Verification items for the finished model (mm, model axes). Face numbers are marked on the shaded views. A direction names the side the tool comes from. Round coordinates to 2 decimals unless told otherwise and drop trailing zeros. Write each loop counter-clockwise with the first axis right and the second up, starting at its lowest first coordinate (ties: lowest second). Pieces come first, ordered by that corner, then holes. Notation, with made-up numbers: M 22,26.25 L 76,26.25 A21 ccw 76,34.25 Z; hole C 12.25,-3 d9. An arc over 180 degrees is marked long. One line per question, with ' | ' between items.
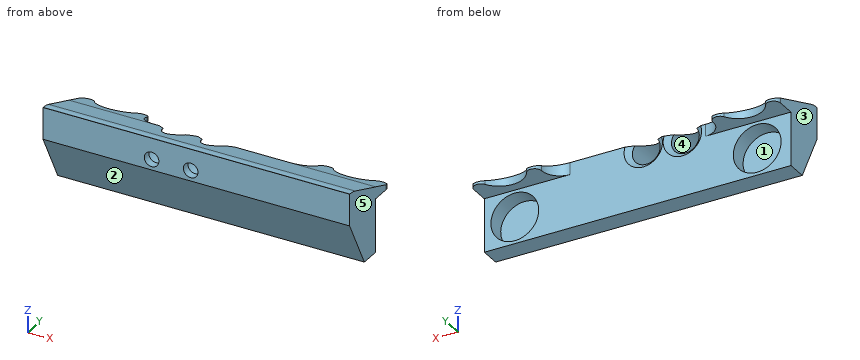
from build123d import *

# Parameters (mm, degrees)
SKETCH1_W               = 115.75
SKETCH1_H               = 30.5
SKETCH1_R               = 2.75
SKETCH1_R_2             = 9.025
BOSS_EXTRUDE1_DEPTH     = 17.25
SKETCH3_R               = 9.025
BOSS_EXTRUDE2_DEPTH     = 10.75
SKETCH4_R               = 5.25
CUT_EXTRUDE1_DEPTH      = 14.25
CUT_EXTRUDE2_DEPTH      = 120.171619944
CUT_EXTRUDE2_DEPTH_BACK = 120.171619944
BOSS_EXTRUDE4_REACH     = 67.617
CHAMFER1_SIZE           = 2


with BuildPart() as part:
    # Sketch1 → Boss-Extrude1 (new body)
    with BuildSketch(Plane(origin=(0, 0, 0), x_dir=(1, 0, 0), z_dir=(0, 1, 0))):
        with Locations((2.125, 7.25)):
            Rectangle(SKETCH1_W, SKETCH1_H)
        with Locations(Location((0, 0, 0), (0, 0, 270))):
            Circle(SKETCH1_R, mode=Mode.SUBTRACT)
        with Locations(Location((-14.75, 0, 0), (0, 0, 270))):
            Circle(SKETCH1_R, mode=Mode.SUBTRACT)
        with Locations(Location((48.5, 12.4, 0), (0, 0, 270))):
            Circle(SKETCH1_R_2, mode=Mode.SUBTRACT)
        with Locations(Location((-43, 12.4, 0), (0, 0, 270))):
            Circle(SKETCH1_R_2, mode=Mode.SUBTRACT)
    extrude(amount=BOSS_EXTRUDE1_DEPTH)

    # Sketch3 → Boss-Extrude2 (add)
    with BuildSketch(Plane.XZ):
        with Locations(Location((48.5, -12.4, 0), (0, 0, 270))):
            Circle(SKETCH3_R)
        with Locations(Location((-43, -12.4, 0), (0, 0, 270))):
            Circle(SKETCH3_R)
    extrude(amount=-BOSS_EXTRUDE2_DEPTH)

    # Sketch4 → Cut-Extrude1 (cut)
    with BuildSketch(Plane(origin=(0, 17.25, 0), x_dir=(1, 0, 0), z_dir=(0, 1, 0))):
        with Locations(Location((-14.75, 0, 0), (0, 0, 270))):
            Circle(SKETCH4_R)
        with Locations(Location((0, 0, 0), (0, 0, 270))):
            Circle(SKETCH4_R)
    extrude(amount=-CUT_EXTRUDE1_DEPTH, mode=Mode.SUBTRACT)

    # Sketch8 → Cut-Extrude2 (cut, two sides: drawn at the far end of the back side and taken through both)
    with BuildSketch(Plane(origin=(60, 0, 0), x_dir=(0, 0, -1), z_dir=(1, 0, 0)).offset(-CUT_EXTRUDE2_DEPTH_BACK)):
        with BuildLine():
            Line((-2.2, 17.25), (-7.34681784, 3.717418611))
            ThreePointArc((-7.34681784, 3.717418611), (-7.835348962, 1.969746414), (-8, 0.162563302))
            Line((-8, 0.162563302), (-8, 17.25))
            Line((-8, 17.25), (-2.2, 17.25))
        make_face()
        Polygon((22.5, 9.75), (4, 0), (22.5, 0), align=None)
    extrude(amount=CUT_EXTRUDE2_DEPTH + CUT_EXTRUDE2_DEPTH_BACK, mode=Mode.SUBTRACT)

    # Boss-Extrude4: up to this plane
    boss_extrude4_end = Plane(origin=(-55.75, 17.25, 2.2), z_dir=(0, -0.35548553095217983, -0.9346817839690934))
    # Sketch7 → Boss-Extrude4 (add, up to the surface)
    with BuildSketch(Plane.XY.offset(-2.3), mode=Mode.PRIVATE) as boss_extrude4_sk1:
        with BuildLine():
            ThreePointArc((39.434120731, 25.3875), (36.45982129, 26.619495167), (34.5, 24.065406335))
            ThreePointArc((34.5, 24.065406335), (32.503813701, 19.246186299), (27.684593665, 17.25))
            Line((27.684593665, 17.25), (60, 17.25))
            Line((60, 17.25), (60, 24.065406335))
            ThreePointArc((60, 24.065406335), (58.04017871, 26.619495167), (55.065879269, 25.3875))
            ThreePointArc((55.065879269, 25.3875), (47.25, 20.875), (39.434120731, 25.3875))
        make_face()
    boss_extrude4_tool1 = split(extrude(boss_extrude4_sk1.sketch, amount=BOSS_EXTRUDE4_REACH, mode=Mode.PRIVATE), bisect_by=boss_extrude4_end, keep=Keep.BOTH, mode=Mode.PRIVATE)
    add(boss_extrude4_tool1.solids().sort_by_distance((46.440425, 20.76167, -2.3))[0])
    # Sketch7 → Boss-Extrude4 (add, up to the surface)
    with BuildSketch(Plane.XY.offset(-2.3), mode=Mode.PRIVATE) as boss_extrude4_sk2:
        with BuildLine():
            ThreePointArc((-30.25, 24.065406335), (-28.253813701, 19.246186299), (-23.434593665, 17.25))
            Line((-23.434593665, 17.25), (-55.75, 17.25))
            Line((-55.75, 17.25), (-55.75, 24.065406335))
            ThreePointArc((-55.75, 24.065406335), (-53.79017871, 26.619495167), (-50.815879269, 25.3875))
            ThreePointArc((-50.815879269, 25.3875), (-43, 20.875), (-35.184120731, 25.3875))
            ThreePointArc((-35.184120731, 25.3875), (-32.20982129, 26.619495167), (-30.25, 24.065406335))
        make_face()
    boss_extrude4_tool2 = split(extrude(boss_extrude4_sk2.sketch, amount=BOSS_EXTRUDE4_REACH, mode=Mode.PRIVATE), bisect_by=boss_extrude4_end, keep=Keep.BOTH, mode=Mode.PRIVATE)
    add(boss_extrude4_tool2.solids().sort_by_distance((-42.190425, 20.76167, -2.3))[0])

    # Chamfer1
    chamfer1_edges = [part.edges().sort_by_distance(p)[0] for p in [
        (0, 17.25, -5.25),
        (-14.75, 17.25, -5.25),
    ]]
    chamfer(chamfer1_edges, length=CHAMFER1_SIZE)


solid = part.part
1. Tool access check on the marked faces 4 and 5. Record the directions out of +Z, -Z, +X, -X, +Y, -Y that give a thin tool (end or side, any length) a straight path to the whole face; none if there is none.
Results:
face 4: +Y | face 5: +Z, -Z, +X, +Y, -Y
2. Mould release check, pull along Z, two halves, no side actions. Record for the marked faces 1, 2 and 3: pulls with the +Z half, pulls with the -Z half, needs draft (parallel to the pull), parting line crosses it, or undercut.
Results:
face 1: undercut | face 2: pulls with the -Z half | face 3: needs draft
3. Section check A-A, the plane y = 13.5. Record the cut outline in (x, z) (3 decimals).
Results:
outline: M -55.75,-22.5 L 60,-22.5 L 60,3.626 L 3.796,3.626 A5.25 cw long -3.796,3.626 L -10.954,3.626 A5.25 cw long -18.546,3.626 L -55.75,3.626 Z; hole C -43,-12.4 d18.05; hole C 48.5,-12.4 d18.05
4. Thickness scan on line 1 (X direction, y = 15.25, z = -12.5); line 2 (X direction, y = 2.3, z = 0); line 3 (Z direction, x = 42.5, y = 14). Record the ranges inside material, lowest first.
Results:
line 1: x = -55.75 to -52.02, -33.98 to 39.48, 57.52 to 60 | line 2: x = -55.75 to -17.5, -12 to -2.75, 2.75 to 60 | line 3: z = -22.5 to -19.14, -5.66 to 3.44
5. Section check C-C, the plane z = -12.4. Record the cut outline in (x, y) (3 decimals), then the cut area to 3 significant figures.
Results:
outline: M -55.75,4.427 L 60,4.427 L 60,17.25 L 57.525,17.25 L 57.525,10.75 L 39.475,10.75 L 39.475,17.25 L -33.975,17.25 L -33.975,10.75 L -52.025,10.75 L -52.025,17.25 L -55.75,17.25 Z | area: 1,250 mm2
6. Section check D-D, the plane x = -43. Record the cut outline in (y, z) (3 decimals).
Results:
outline: M 0,-4 L 9.75,-22.5 L 17.25,-22.5 L 17.25,-21.425 L 10.75,-21.425 L 10.75,-3.375 L 17.25,-3.375 L 17.25,-2.3 L 20.875,-2.3 L 20.875,0.821 L 3.717,7.347 A10 ccw 0.163,8 L 0,8 Z
7. Section check B-B, the plane x = -14.75. Record the cut outline in (y, z), then the cut area to 3 significant figures.
Results:
outline: M 0,-4 L 9.75,-22.5 L 17.25,-22.5 L 17.25,-7.25 L 15.25,-5.25 L 3,-5.25 L 3,-2.75 L 0,-2.75 Z; M 0,2.75 L 3,2.75 L 3,5.25 L 9.23,5.25 L 3.72,7.35 A10 ccw 0.16,8 L 0,8 Z | area: 236 mm2
8. Go/stop test with flat-tipped pins: P1, Ø2, axis at x = -34, y = 6, coming from the +Z side; P2, Ø3, axis at x = -38.5, y = 23.5, coming from the -Z side; P3, Ø6, axis at x = 4, z = -8, coming from the -Y side. Record where each tip stops, or that it passes through.
Results:
P1: stops at z = 6.86 | P2: stops at z = -2.3 | P3: stops at y = 0.53
